Design review of the part built by this model. Coordinates are the model's own, in mm. Coordinates: 2 decimals unless noted, no trailing zeros. Write each loop counter-clockwise with the first axis right and the second up, starting at its lowest first coordinate (ties: lowest second). Pieces come first, ordered by that corner, then holes.
Q1. For probe 1 along Z at (x, y) = (-1.25, 22.5); probe 2 along X at (y, z) = (32.5, -3), list the stretches that pass through material, from the lowest coordinate up.
Q2. Take a section at B-B (z = 0). Give the boundary of the cut face in (x, y).
Q3. Take a section at A-A (x = 0). Give the boundary of the cut face in (y, z), and give its area (3 significant figures).
Q4. Insertion check: pin 1 (0.9 mm diameter, centred on x = 0.5, y = 79, fed in from +Z). The pin has a flat end and moves straight along its axis. Give the tip position at first contact, or say it passes through.
```python
from build123d import *

# Parameters (mm, degrees)
SKETCH1_R           = 1
BOSS_EXTRUDE1_DEPTH = 110


with BuildPart() as part:
    # Sketch1 → Boss-Extrude1 (new body)
    with BuildSketch(Plane(origin=(0, 0, 0), x_dir=(1, 0, 0), z_dir=(0, 1, 0))):
        with BuildLine():
            Line((1.25, 6), (6, 6))
            Line((6, 6), (6, 1.25))
            ThreePointArc((6, 1.25), (5.926776695, 1.073223305), (5.75, 1))
            Line((5.75, 1), (4.75, 1))
            ThreePointArc((4.75, 1), (4.573223305, 1.073223305), (4.5, 1.25))
            Line((4.5, 1.25), (4.5, 2.973453617))
            ThreePointArc((4.5, 2.973453617), (4.380872479, 3.151740551), (4.170568701, 3.109908529))
            Line((4.170568701, 3.109908529), (2.5, 1.439339828))
            Line((2.5, 1.439339828), (2.5, -1.439339828))
            Line((2.5, -1.439339828), (4.170568701, -3.109908529))
            ThreePointArc((4.170568701, -3.109908529), (4.380872479, -3.151740551), (4.5, -2.973453617))
            Line((4.5, -2.973453617), (4.5, -1.25))
            ThreePointArc((4.5, -1.25), (4.573223305, -1.073223305), (4.75, -1))
            Line((4.75, -1), (5.75, -1))
            ThreePointArc((5.75, -1), (5.926776695, -1.073223305), (6, -1.25))
            Line((6, -1.25), (6, -6))
            Line((6, -6), (1.25, -6))
            ThreePointArc((1.25, -6), (1.073223305, -5.926776695), (1, -5.75))
            Line((1, -5.75), (1, -4.75))
            ThreePointArc((1, -4.75), (1.073223305, -4.573223305), (1.25, -4.5))
            Line((1.25, -4.5), (2.973453617, -4.5))
            ThreePointArc((2.973453617, -4.5), (3.151740551, -4.380872479), (3.109908529, -4.170568701))
            Line((3.109908529, -4.170568701), (1.439339828, -2.5))
            Line((1.439339828, -2.5), (-1.439339828, -2.5))
            Line((-1.439339828, -2.5), (-3.109908529, -4.170568701))
            ThreePointArc((-3.109908529, -4.170568701), (-3.151740551, -4.380872479), (-2.973453617, -4.5))
            Line((-2.973453617, -4.5), (-1.25, -4.5))
            ThreePointArc((-1.25, -4.5), (-1.073223305, -4.573223305), (-1, -4.75))
            Line((-1, -4.75), (-1, -5.75))
            ThreePointArc((-1, -5.75), (-1.073223305, -5.926776695), (-1.25, -6))
            Line((-1.25, -6), (-6, -6))
            Line((-6, -6), (-6, -1.25))
            ThreePointArc((-6, -1.25), (-5.926776695, -1.073223305), (-5.75, -1))
            Line((-5.75, -1), (-4.75, -1))
            ThreePointArc((-4.75, -1), (-4.573223305, -1.073223305), (-4.5, -1.25))
            Line((-4.5, -1.25), (-4.5, -2.973453617))
            ThreePointArc((-4.5, -2.973453617), (-4.380872479, -3.151740551), (-4.170568701, -3.109908529))
            Line((-4.170568701, -3.109908529), (-2.5, -1.439339828))
            Line((-2.5, -1.439339828), (-2.5, 1.439339828))
            Line((-2.5, 1.439339828), (-4.170568701, 3.109908529))
            ThreePointArc((-4.170568701, 3.109908529), (-4.380872479, 3.151740551), (-4.5, 2.973453617))
            Line((-4.5, 2.973453617), (-4.5, 1.25))
            ThreePointArc((-4.5, 1.25), (-4.573223305, 1.073223305), (-4.75, 1))
            Line((-4.75, 1), (-5.75, 1))
            ThreePointArc((-5.75, 1), (-5.926776695, 1.073223305), (-6, 1.25))
            Line((-6, 1.25), (-6, 6))
            Line((-6, 6), (-1.25, 6))
            ThreePointArc((-1.25, 6), (-1.073223305, 5.926776695), (-1, 5.75))
            Line((-1, 5.75), (-1, 4.75))
            ThreePointArc((-1, 4.75), (-1.073223305, 4.573223305), (-1.25, 4.5))
            Line((-1.25, 4.5), (-2.973453617, 4.5))
            ThreePointArc((-2.973453617, 4.5), (-3.151740551, 4.380872479), (-3.109908529, 4.170568701))
            Line((-3.109908529, 4.170568701), (-1.439339828, 2.5))
            Line((-1.439339828, 2.5), (1.439339828, 2.5))
            Line((1.439339828, 2.5), (3.109908529, 4.170568701))
            ThreePointArc((3.109908529, 4.170568701), (3.151740551, 4.380872479), (2.973453617, 4.5))
            Line((2.973453617, 4.5), (1.25, 4.5))
            ThreePointArc((1.25, 4.5), (1.073223305, 4.573223305), (1, 4.75))
            Line((1, 4.75), (1, 5.75))
            ThreePointArc((1, 5.75), (1.073223305, 5.926776695), (1.25, 6))
        make_face()
        with Locations(Location((0, 0, 0), (0, 0, 270))):
            Circle(SKETCH1_R, mode=Mode.SUBTRACT)
    extrude(amount=BOSS_EXTRUDE1_DEPTH)


solid = part.part
```
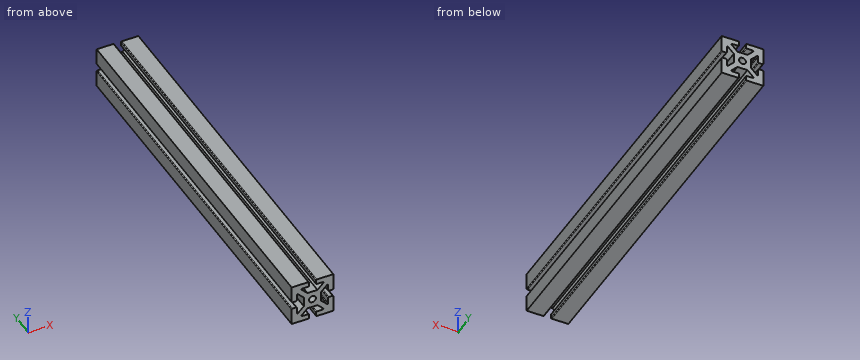
Response:
1. probe 1: z = -6 to -4.5, -2.5 to 2.5, 4.5 to 6
1. probe 2: x = -6 to -4.5, -4.06 to -1.94, 1.94 to 4.06, 4.5 to 6
2. outline: (-2.5, 0) - (-1, 0) - (-1, 110) - (-2.5, 110) - close; (1, 0) - (2.5, 0) - (2.5, 110) - (1, 110) - close
3. outline: (0, -2.5) - (110, -2.5) - (110, -1) - (0, -1) - close; (0, 1) - (110, 1) - (110, 2.5) - (0, 2.5) - close
3. area: 330 mm2
4. pin 1: stops at z = 2.5
